Could you check a few things on this drawing? It's one solid part, dimensions in mm from its lowest x, y, z. A direction names the side the tool comes from. Give positions to 0.01 mm unless a question says otherwise; leave off trailing zeros. Loops run counter-clockwise (first coordinate to the right, second up) from the corner with the lowest first, then second, coordinate; pieces in that order, holes last. Notation, with made-up numbers: (65.5, 84.25) - (95.5, 84.25) arc R17 ccw to (95.5, 101.25) - close; hole circle Ø5 at (2, 85). An arc over 180 degrees is marked (long way). Write each question's results on one line, items separated by ' | '. Start each with the question number.
(1) I need wall thicknesses on line 1 (Y direction, x = 28.5, z = 8.5) (1 decimal); line 2 (Z direction, x = 68, y = 6.5); line 3 (Y direction, x = 96, z = 3.25) (1 decimal). Which ranges of each line are inside material? Lowest first, please.
(2) Suppose I cut it at C-C (x = 37). Please give me the cut outline in (y, z) (1 decimal), and give its area (3 significant figures).
(3) On a 3-axis mill with a long thin cutter (end or side, diameter ignored), from which of +Z, -Z, +X, -X, +Y, -Y can I reach the whole of each face in a straight line? I mean the marked faces 1, 2 and 3. Say none if no direction works.
(4) For pin 1 (3 mm diameter, centred on x = 69, y = 22.5, fed in from +Z); pin 2 (5 mm diameter, centred on x = 70.5, z = 20.5, fed in from -Y) (1 decimal); pin 3 (8 mm diameter, centred on x = 47.5, z = 9.5, fed in from +Y) (1 decimal), each with a flat end and sliding along its axis, tell me the tip position at first contact or that it passes through.
(5) Suppose I cut it at A-A (y = 18). Please give me the cut outline in (x, z), and give its area (3 significant figures).
(6) If we mould it in two halves opening along X, with no side actions, what happens to the marked faces 4 and 5? For each: released by +X, released by -X, zero draft, split by the parting line, or undercut.
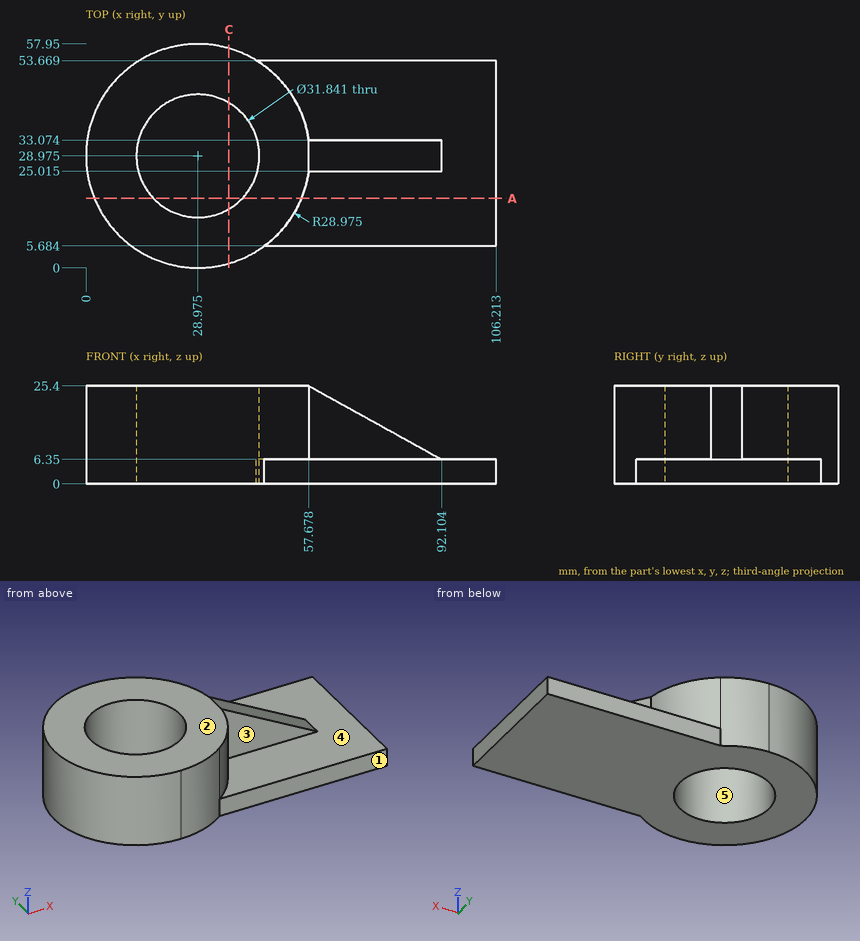
Output values:
1) line 1: 0 to 13.1, 44.9 to 57.9 | line 2: 0 to 6.35 | line 3: 5.7 to 53.7
2) outline: (1.1, 0) - (15.2, 0) - (15.2, 25.4) - (1.1, 25.4) - close; (42.7, 0) - (56.8, 0) - (56.8, 25.4) - (42.7, 25.4) - close | area: 716 mm2
3) face 1: +Z, -Z, +X, -Y | face 2: +Z, +X, -X, +Y, -Y | face 3: +Z, +X, -Y
4) pin 1: z = 6.35 | pin 2: y = 25 | pin 3: y = 54
5) outline: (2.16, 0) - (17.44, 0) - (17.44, 25.4) - (2.16, 25.4) - close; (40.51, 0) - (106.21, 0) - (106.21, 6.35) - (55.79, 6.35) - (55.79, 25.4) - (40.51, 25.4) - close | area: 1,100 mm2
6) face 4: zero draft | face 5: undercut
